For this review, take the finished solid that the model builds, in its own axes (mm). Round coordinates to 2 decimals unless told otherwise and drop trailing zeros. Write each loop counter-clockwise with the first axis right and the second up, starting at its lowest first coordinate (ties: lowest second). Pieces come first, ordered by that corner, then holes.
from build123d import *

# Parameters (mm, degrees)
SKETCH3_W           = 75
SKETCH3_H           = 75
SKETCH3_W_2         = 55
SKETCH3_H_2         = 55
BOSS_EXTRUDE2_DEPTH = 826.205


with BuildPart() as part:
    # Sketch3 → Boss-Extrude2 (new, along a direction that is not the sketch's normal)
    with BuildSketch(Plane(origin=(0, 0, 0), x_dir=(1, 0, 0), z_dir=(0, 1, 0))):
        Rectangle(SKETCH3_W, SKETCH3_H)
        Rectangle(SKETCH3_W_2, SKETCH3_H_2, mode=Mode.SUBTRACT)
    extrude(amount=-BOSS_EXTRUDE2_DEPTH, dir=(-0.7960914026765946, 0.6051764028648275, 0))


solid = part.part
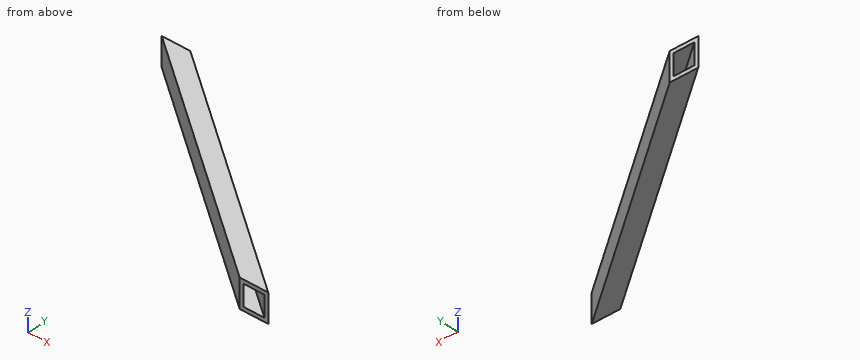
(1) For pin 1 Ø10 at (y, z) = (-148, -25.5) entering from -X; pin 2 Ø1 at (y, z) = (-414.5, -11) entering from -X; pin 3 Ø12 at (y, z) = (-410, -29) entering from +X, all flat-tipped, find the tip position at first contact; note any pin that passes through.
Geometry check:
pin 1: stops at x = 150.61
pin 2: stops at x = 507.1
pin 3: stops at x = 584.74
(2) We need section B-B, the plane x = 351. Give the boundary of the cut face in (y, z).
Geometry check:
outline: (-295.33, -37.5) - (-238.32, -37.5) - (-238.32, 37.5) - (-295.33, 37.5) - close; hole (-287.73, -27.5) - (-245.92, -27.5) - (-245.92, 27.5) - (-287.73, 27.5) - close
(3) For line 1 along Z through (x, y) = (409, -327.5); line 2 along X through (y, z) = (-464, -14); line 3 along Y through (x, z) = (116, -7), list the stretches that pass through material, from the lowest coordinate up.
Geometry check:
line 1: z = -37.5 to -27.5, 27.5 to 37.5
line 2: x = 572.88 to 582.88, 637.88 to 647.88
line 3: y = -116.69 to -109.09, -67.28 to -59.67
(4) We need section D-D, the plane x = 12.5. Give the boundary of the cut face in (y, z), and give its area (3 significant figures).
Geometry check:
outline: (-38.01, -37.5) - (0, -37.5) - (0, -27.5) - (-30.41, -27.5) - (-30.41, 27.5) - (0, 27.5) - (0, 37.5) - (-38.01, 37.5) - close
area: 1,180 mm2
(5) We need section A-A, the plane z = 11. Give the boundary of the cut face in (x, y).
Geometry check:
outline: (-37.5, 0) - (620.23, -500) - (630.23, -500) - (-27.5, 0) - close; (27.5, 0) - (685.23, -500) - (695.23, -500) - (37.5, 0) - close
(6) We need section C-C, the plane y = -175. Give the boundary of the cut face in (x, z).
Geometry check:
outline: (192.71, -37.5) - (267.71, -37.5) - (267.71, 37.5) - (192.71, 37.5) - close; hole (202.71, -27.5) - (257.71, -27.5) - (257.71, 27.5) - (202.71, 27.5) - close
